```python
from build123d import *

# Parameters (mm, degrees)
ESQUISSE2_W             = 300
ESQUISSE2_H             = 300
BOSS_EXTRU_1_DEPTH      = 3
ESQUISSE3_W             = 50
ESQUISSE3_H             = 2.95
ESQUISSE3_W_2           = 2.95
ESQUISSE3_H_2           = 50
ENL_V_MAT_EXTRU_2_DEPTH = 6
ESQUISSE5_W             = 2.95
ESQUISSE5_H             = 50
ESQUISSE5_W_2           = 50
ESQUISSE5_H_2           = 2.95
ENL_V_MAT_EXTRU_3_DEPTH = 6
ENL_V_MAT_EXTRU_4_DEPTH = 6
SYM_TRIE2_COPY_1_DEPTH  = 6
SYM_TRIE2_COPY_2_DEPTH  = 6


with BuildPart() as part:
    # Esquisse2 → Boss.-Extru.1 (new body)
    with BuildSketch(Plane.XY):
        Rectangle(ESQUISSE2_W, ESQUISSE2_H)
    extrude(amount=BOSS_EXTRU_1_DEPTH)

    # Esquisse3 → Enlèv. mat.-Extru.2 (cut)
    with BuildSketch(Plane.XY.offset(3)):
        with Locations((-95, 138.525)):
            Rectangle(ESQUISSE3_W, ESQUISSE3_H)
        with Locations((-138.525, 95)):
            Rectangle(ESQUISSE3_W_2, ESQUISSE3_H_2)
    extrude(amount=-ENL_V_MAT_EXTRU_2_DEPTH, mode=Mode.SUBTRACT)

    # Esquisse5 → Enlèv. mat.-Extru.3 (cut)
    with BuildSketch(Plane(origin=(0, 0, 0), x_dir=(-1, 0, 0), z_dir=(0, 0, -1))):
        with Locations((138.525, -95)):
            Rectangle(ESQUISSE5_W, ESQUISSE5_H)
        with Locations((95, -138.525)):
            Rectangle(ESQUISSE5_W_2, ESQUISSE5_H_2)
        with Locations((-95, -138.525)):
            Rectangle(ESQUISSE5_W_2, ESQUISSE5_H_2)
        with Locations((-138.525, -95)):
            Rectangle(ESQUISSE5_W, ESQUISSE5_H)
        with Locations((-138.525, 95)):
            Rectangle(ESQUISSE5_W, ESQUISSE5_H)
        with Locations((-95, 138.525)):
            Rectangle(ESQUISSE5_W_2, ESQUISSE5_H_2)
    extrude(amount=-ENL_V_MAT_EXTRU_3_DEPTH, mode=Mode.SUBTRACT)

    # Esquisse6 → Enlèv. mat.-Extru.4 (cut)
    with BuildSketch(Plane(origin=(0, 0, 0), x_dir=(-1, 0, 0), z_dir=(0, 0, -1))):
        with BuildLine():
            Line((150, 6.25), (143.325317547, 6.25))
            ThreePointArc((143.325317547, 6.25), (120, 0), (143.325317547, -6.25))
            Line((143.325317547, -6.25), (150, -6.25))
            Line((150, -6.25), (150, 6.25))
        make_face()
        with BuildLine():
            Line((-6.25, -150), (6.25, -150))
            Line((6.25, -150), (6.25, -143.325317547))
            ThreePointArc((6.25, -143.325317547), (0, -120), (-6.25, -143.325317547))
            Line((-6.25, -143.325317547), (-6.25, -150))
        make_face()
    enl_v_mat_extru_4 = extrude(amount=-ENL_V_MAT_EXTRU_4_DEPTH, mode=Mode.SUBTRACT)

    # Symétrie1: Enlèv. mat.-Extru.4 across plane
    add(enl_v_mat_extru_4.mirror(Plane(origin=(0, 0, 0), x_dir=(0, 0, 1), z_dir=(1, 0, 0))), mode=Mode.SUBTRACT)

    # Symétrie2 copy 1 sketch → Symétrie2 copy 1 (cut)
    with BuildSketch(Plane(origin=(0, 0, 0), x_dir=(1, 0, 0), z_dir=(0, 0, -1))):
        with BuildLine():
            Line((150, 6.25), (143.325317547, 6.25))
            ThreePointArc((143.325317547, 6.25), (120, 0), (143.325317547, -6.25))
            Line((143.325317547, -6.25), (150, -6.25))
            Line((150, -6.25), (150, 6.25))
        make_face()
        with BuildLine():
            Line((-6.25, -150), (6.25, -150))
            Line((6.25, -150), (6.25, -143.325317547))
            ThreePointArc((6.25, -143.325317547), (0, -120), (-6.25, -143.325317547))
            Line((-6.25, -143.325317547), (-6.25, -150))
        make_face()
    extrude(amount=-SYM_TRIE2_COPY_1_DEPTH, mode=Mode.SUBTRACT)

    # Symétrie2 copy 2 sketch → Symétrie2 copy 2 (cut)
    with BuildSketch(Plane(origin=(0, 0, 0), x_dir=(-1, 0, 0), z_dir=(0, 0, -1))):
        with BuildLine():
            Line((150, -6.25), (143.325317547, -6.25))
            ThreePointArc((143.325317547, -6.25), (120, 0), (143.325317547, 6.25))
            Line((143.325317547, 6.25), (150, 6.25))
            Line((150, 6.25), (150, -6.25))
        make_face()
        with BuildLine():
            Line((-6.25, 150), (6.25, 150))
            Line((6.25, 150), (6.25, 143.325317547))
            ThreePointArc((6.25, 143.325317547), (0, 120), (-6.25, 143.325317547))
            Line((-6.25, 143.325317547), (-6.25, 150))
        make_face()
    extrude(amount=-SYM_TRIE2_COPY_2_DEPTH, mode=Mode.SUBTRACT)


solid = part.part
```
Read the model definition and answer for the solid it produces. Units are mm, in the model's axes. Give positions to 0.01 mm unless a question says otherwise; leave off trailing zeros. Order: outer loops, then holes, each group sorted by start corner. A loop starts at its lowest first (then second) coordinate and runs counter-clockwise, first axis right, second up. Notation, with made-up numbers: (71, -19) -> (102, -19) arc R18 ccw to (102, 5) -> close; hole circle Ø9 at (31.25, 12). An arc over 180 degrees is marked (long way). One line per item, written item: value. Start each with the question number.
(1) The part is cut by section C-C (x = 79.5). Determine the outline of the cut face in (y, z).
(2) Straight lines are drawn through the part: L1, parallel to X at y = -89, z = 0.85; L2, parallel to Y at x = -11, z = 0.65; L3, parallel to X at y = 132.5, z = 2.05. For each, find the intervals that lie inside material, in ascending order.
(3) For a pull along X with two mould halves and no side action, classify faces 1 (the flat face through (-2, 2, 3)), 2 (the cylindrical face through (0, -120, 1)), 3 (the cylindrical face through (0, 120, 1)) as released by +X, released by -X, zero draft, split by the parting line, or undercut.
(4) A flat-ended cylindrical pin translates along its axis: P1, Ø15, axis at x = -132.5, y = 0, coming from the -Z side. Find the tip coordinate at first contact, or state that the pin passes through.
(5) The part is cut by section D-D (z = 1.45). State how many separate pieces and enclosed holes the cut face has, and give its area (3 significant figures).
(6) The part is cut by section A-A (x = 132.5). Determine the outline of the cut face in (y, z), and give its area (3 significant figures).
Taken from the geometry:
1. outline: (-150, 0) -> (-140, 0) -> (-140, 3) -> (-150, 3) -> close; (-137.05, 0) -> (137.05, 0) -> (137.05, 3) -> (-137.05, 3) -> close; (140, 0) -> (150, 0) -> (150, 3) -> (140, 3) -> close
2. L1: -150 to -140, -137.05 to 137.05, 140 to 150
2. L2: -150 to -138.44, -126.56 to 126.56, 138.44 to 150
2. L3: -150 to -12.5, 12.5 to 150
3. face 1: zero draft
3. face 2: undercut
3. face 3: undercut
4. P1: through
5. separate pieces: 1
5. enclosed holes: 8
5. area: 86,600 mm^2
6. outline: (-150, 0) -> (-12.5, 0) -> (-12.5, 3) -> (-150, 3) -> close; (12.5, 0) -> (150, 0) -> (150, 3) -> (12.5, 3) -> close
6. area: 825 mm^2
